Source: three-view drawing plus pictorial views. Frame: mm from the lowest corner of the part. A direction names the side the tool comes from. Round coordinates to 2 decimals unless told otherwise and drop trailing zeros. Order: outer loops, then holes, each group sorted by start corner. A loop starts at its lowest first (then second) coordinate and runs counter-clockwise, first axis right, second up. Notation, with made-up numbers: (42.5, 86) -> (59.5, 86) arc R23 cw to (59.5, 124) -> close; hole circle Ø3 at (1, 8). An arc over 180 degrees is marked (long way). Answer as CSV lines item,"result".
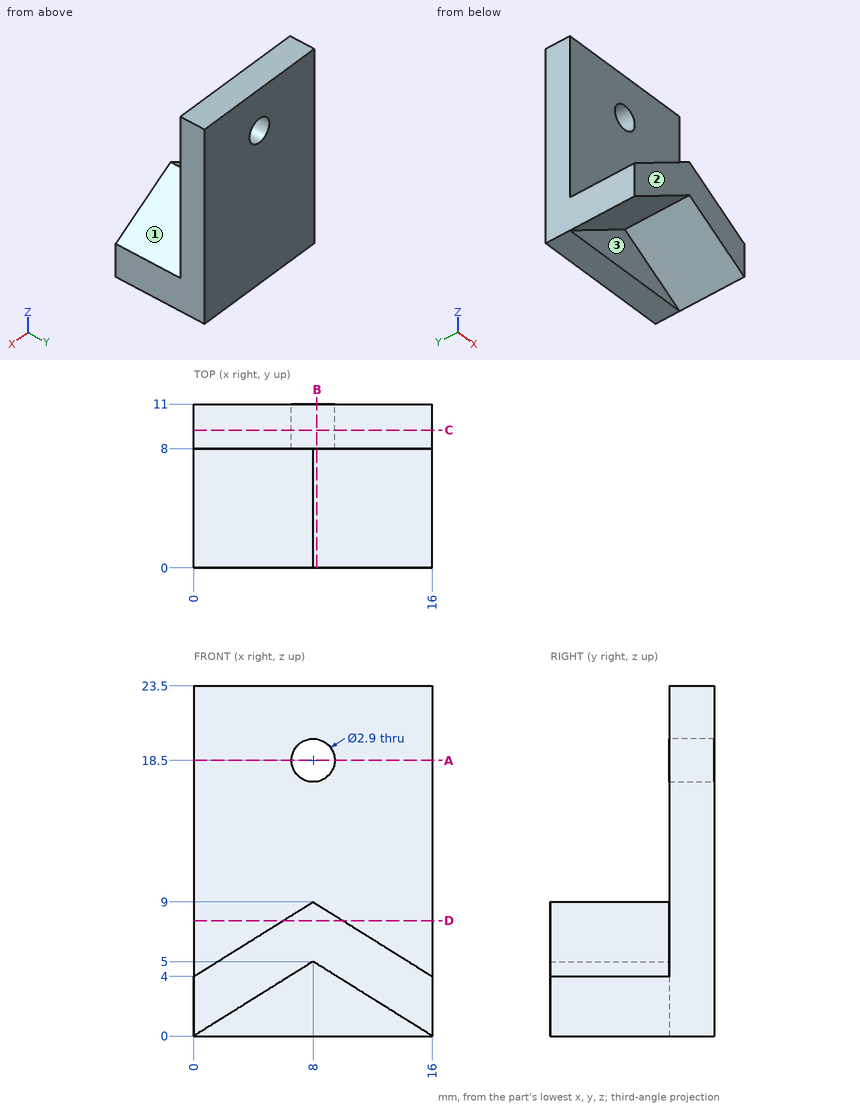
1. Section query D-D on z = 7.75. Return loops of the section in (x, y), and give its area (3 significant figures).
Results below:
outline,"(0, 8) -> (6, 8) -> (6, 0) -> (10, 0) -> (10, 8) -> (16, 8) -> (16, 11) -> (0, 11) -> close"
area,"80.0 mm2"
2. Section query C-C on y = 9.25. Return loops of the section in (x, z), and give its area (3 significant figures).
Results below:
outline,"(0, 0) -> (16, 0) -> (16, 23.5) -> (0, 23.5) -> close; hole circle Ø2.9 at (8, 18.5)"
area,"369 mm2"
3. Line query: L1, parallel to X at y = 9.8, z = 18.5; L2, parallel to Y at x = 9.75, z = 19.5; L3, parallel to X at y = 5.5, z = 4.5. Output: solid intervals per line, ascending. Write a range as [from, to].
Results below:
L1,"[0, 6.55], [9.45, 16]"
L2,"[8, 11]"
L3,"[0.8, 7.2], [8.8, 15.2]"
4. Section query A-A on z = 18.5. Return loops of the section in (x, y), and give its area (3 significant figures).
Results below:
outline,"(0, 8) -> (6.55, 8) -> (6.55, 11) -> (0, 11) -> close; (9.45, 8) -> (16, 8) -> (16, 11) -> (9.45, 11) -> close"
area,"39.3 mm2"
5. Reachability of the marked faces 1, 2 and 3 from +Z, -Z, +X, -X, +Y, -Y: full face, straight path, thin tool, end or side. Return the list, or none.
Results below:
face 1,"+Z, +X, -Y"
face 2,"+Z, -Z, +X, -X, -Y"
face 3,"-Z, -Y"
6. Pin query (flat end, axial travel): pin 1 (2.5 mm diameter, centred on x = 7.5, z = 1.5, fed in from -Y); pin 2 (2.5 mm diameter, centred on x = 8, z = 18.5, fed in from -Y); pin 3 (5 mm diameter, centred on x = 9.5, y = 4.5, fed in from -Z). Return the tip coordinate at first contact, or that it passes through.
Results below:
pin 1,"y = 8"
pin 2,"through"
pin 3,"z = 2.5"
7. Section query B-B on x = 8.25. Return loops of the section in (y, z), and give its area (3 significant figures).
Results below:
outline,"(0, 4.84) -> (8, 4.84) -> (8, 0) -> (11, 0) -> (11, 17.07) -> (8, 17.07) -> (8, 8.84) -> (0, 8.84) -> close; (8, 19.93) -> (11, 19.93) -> (11, 23.5) -> (8, 23.5) -> close"
area,"93.9 mm2"
